from build123d import *

# Parameters (mm, degrees)
SKETCH1_W           = 30
SKETCH1_H           = 50
SKETCH1_R           = 1.25
BOSS_EXTRUDE1_DEPTH = 5
FILLET1_R           = 5
BOSS_EXTRUDE2_DEPTH = 2


with BuildPart() as part:
    # Sketch1 → Boss-Extrude1 (new body)
    with BuildSketch(Plane(origin=(0, 0, 0), x_dir=(1, 0, 0), z_dir=(0, 1, 0))):
        with Locations((3.5, 0)):
            Rectangle(SKETCH1_W, SKETCH1_H)
        with Locations(Location((0, 0, 0), (0, 0, 270))):
            Circle(SKETCH1_R, mode=Mode.SUBTRACT)
        with Locations(Location((0, 7, 0), (0, 0, 270))):
            Circle(SKETCH1_R, mode=Mode.SUBTRACT)
        with Locations(Location((7, 0, 0), (0, 0, 270))):
            Circle(SKETCH1_R, mode=Mode.SUBTRACT)
        with Locations(Location((0, -7, 0), (0, 0, 270))):
            Circle(SKETCH1_R, mode=Mode.SUBTRACT)
    extrude(amount=BOSS_EXTRUDE1_DEPTH)

    # Fillet1
    fillet1_edges = [part.edges().sort_by_distance(p)[0] for p in [
        (-11.5, 2.5, -25),
        (18.5, 2.5, -25),
        (18.5, 2.5, 25),
        (-11.5, 2.5, 25),
    ]]
    fillet(fillet1_edges, radius=FILLET1_R)

    # Sketch2 → Boss-Extrude2 (add)
    with BuildSketch(Plane(origin=(0, 5, 0), x_dir=(1, 0, 0), z_dir=(0, 1, 0))):
        Polygon((11.600813037, 18.856220698), (11.600813037, 8.856220698), (13.600813037, 8.856220698), (13.600813037, 18.856220698), (16.600813037, 18.856220698), (12.600813037, 22.856220698), (8.600813037, 18.856220698), align=None)
    extrude(amount=BOSS_EXTRUDE2_DEPTH)


solid = part.part
Geometry check sheet. Reference: the model listing, model coordinates, mm. A direction names the side the tool comes from. Round coordinates to 2 decimals unless told otherwise and drop trailing zeros. Write each loop counter-clockwise with the first axis right and the second up, starting at its lowest first coordinate (ties: lowest second). Pieces come first, ordered by that corner, then holes. Notation, with made-up numbers: (32.5, 24) -> (39.5, 24) arc R15 ccw to (39.5, 29) -> close; hole circle Ø11 at (69.5, 16.25). An arc over 180 degrees is marked (long way). One line per item, written item: value. Start each with the question number.
(1) Cross-section at D-D, the plane x = 7.75. Record the cut outline in (y, z), and give its area (3 significant figures).
(2) Cross-section at B-B, the plane z = 7. Record the cut outline in (x, y).
(3) Cross-section at A-A, the plane x = 0. Record the cut outline in (y, z).
(4) Scan lines: line 1 (X direction, y = 3.15, z = 0); line 2 (X direction, y = 2.85, z = 7); line 3 (Y direction, x = 5.5, z = 9.5). Record each from-to range of solid material in increasing order. Write a range as [from, to].
(5) Draft check along Z on faces 6 (the cylindrical face through (-1.22, 2.46, -0.27)), 7 (the cylindrical face through (0.05, 2.46, 5.75)), 8 (the flat face through (15, 6, -18.856)), 9 (the cylindrical face through (17, 2.54, -23.57)). Enter one of: +Z half, -Z half, draft (parallel to the pull), parting line (faces both ways), or undercut.
(6) Go/stop test with flat-tipped pins: pin 1 Ø2 at (x, z) = (7, 0) entering from +Y; pin 2 Ø12 at (x, z) = (8.5, 20) entering from +Y; pin 3 Ø2 at (x, y) = (12.5, 6.5) entering from +Z; pin 4 Ø0.6 at (x, y) = (15.5, 6) entering from +Z. Record where each tip stops, or that it passes through.
(7) Cross-section at C-C, the plane z = 0. Record the cut outline in (x, y).
(8) Access from +Z, -Z, +X, -X, +Y, -Y to the whole of each face (thin tool, end or side, straight path). Record for faces 1 (the flat face through (11.601, 6, -14)), 2 (the flat face through (3, 2, 25)), 3 (the flat face through (18.5, 2, 0)), 4 (the flat face through (13, 6, -8.856)), 5 (the flat face through (10.629, 5.986, -20.884)).
Answer:
1. outline: (0, -25) -> (5, -25) -> (5, -1) -> (0, -1) -> close; (0, 1) -> (5, 1) -> (5, 25) -> (0, 25) -> close
1. area: 240 mm²
2. outline: (-11.5, 0) -> (-1.25, 0) -> (-1.25, 5) -> (-11.5, 5) -> close; (1.25, 0) -> (18.5, 0) -> (18.5, 5) -> (1.25, 5) -> close
3. outline: (0, -25) -> (5, -25) -> (5, -8.25) -> (0, -8.25) -> close; (0, -5.75) -> (5, -5.75) -> (5, -1.25) -> (0, -1.25) -> close; (0, 1.25) -> (5, 1.25) -> (5, 5.75) -> (0, 5.75) -> close; (0, 8.25) -> (5, 8.25) -> (5, 25) -> (0, 25) -> close
4. line 1: [-11.5, -1.25], [1.25, 5.75], [8.25, 18.5]
4. line 2: [-11.5, -1.25], [1.25, 18.5]
4. line 3: [0, 5]
5. face 6: undercut
5. face 7: undercut
5. face 8: +Z half
5. face 9: -Z half
6. pin 1: through
6. pin 2: y = 5
6. pin 3: z = -8.86
6. pin 4: z = -18.86
7. outline: (-11.5, 0) -> (-1.25, 0) -> (-1.25, 5) -> (-11.5, 5) -> close; (1.25, 0) -> (5.75, 0) -> (5.75, 5) -> (1.25, 5) -> close; (8.25, 0) -> (18.5, 0) -> (18.5, 5) -> (8.25, 5) -> close
8. face 1: +Z, -X, +Y
8. face 2: +Z, +X, -X, +Y, -Y
8. face 3: +Z, -Z, +X, +Y, -Y
8. face 4: +Z, +X, -X, +Y
8. face 5: -Z, -X, +Y
